from build123d import *

# Parameters (mm, degrees)
F_1_4_20_TAPPED_HOLE1_D     = 5.1054
F_1_4_20_TAPPED_HOLE1_DEPTH = 16.51
F_1_4_20_TAPPED_HOLE1_TIP   = 1.533816902
CUT_EXTRUDE1_DEPTH          = 9.525


with BuildPart() as part:
    # Sketch1 → Revolve2 (revolve)
    with BuildSketch(Plane(origin=(0, 0, 0), x_dir=(0, 0, -1), z_dir=(1, 0, 0)), mode=Mode.PRIVATE) as revolve2_sk:
        Polygon((38.1, 6.2865), (0, 6.2865), (0, 0), (82.55, 0), (82.55, 6.35), (44.45, 6.35), (44.45, 11.43), (38.1, 11.43), align=None)
    revolve(revolve2_sk.sketch.rotate(Axis((0, 0, 0), (0, 0, -1)), 90), axis=Axis((0, 0, 0), (0, 0, -1)))

    # 1/4-20 Tapped Hole1
    with Locations(Plane(origin=(0, 0, -82.55), x_dir=(-1, 0, 0), z_dir=(0, 0, -1))):
        with Locations((0, 0)):
            Hole(F_1_4_20_TAPPED_HOLE1_D / 2, depth=F_1_4_20_TAPPED_HOLE1_DEPTH)
            with Locations((0, 0, -(F_1_4_20_TAPPED_HOLE1_DEPTH + F_1_4_20_TAPPED_HOLE1_TIP / 2))):  # 118° drill point
                Cone(0, F_1_4_20_TAPPED_HOLE1_D / 2, F_1_4_20_TAPPED_HOLE1_TIP, mode=Mode.SUBTRACT)

    # Sketch4 → Cut-Extrude1 (cut)
    with BuildSketch(Plane.XY):
        with BuildLine():
            ThreePointArc((2.9407768, 5.55625), (0, 6.2865), (-2.9407768, 5.55625))
            Line((-2.9407768, 5.55625), (2.9407768, 5.55625))
        make_face()
        with BuildLine():
            ThreePointArc((6.28224205, 0.231337584), (5.444268701, 3.14325), (3.34146525, 5.324912416))
            Line((3.34146525, 5.324912416), (6.28224205, 0.231337584))
        make_face()
        with BuildLine():
            Line((6.28224205, -0.231337584), (3.34146525, -5.324912416))
            ThreePointArc((3.34146525, -5.324912416), (5.444268701, -3.14325), (6.28224205, -0.231337584))
        make_face()
        with BuildLine():
            Line((2.9407768, -5.55625), (-2.9407768, -5.55625))
            ThreePointArc((-2.9407768, -5.55625), (0, -6.2865), (2.9407768, -5.55625))
        make_face()
        with BuildLine():
            Line((-3.34146525, -5.324912416), (-6.28224205, -0.231337584))
            ThreePointArc((-6.28224205, -0.231337584), (-5.444268701, -3.14325), (-3.34146525, -5.324912416))
        make_face()
        with BuildLine():
            ThreePointArc((-3.34146525, 5.324912416), (-5.444268701, 3.14325), (-6.28224205, 0.231337584))
            Line((-6.28224205, 0.231337584), (-3.34146525, 5.324912416))
        make_face()
    extrude(amount=-CUT_EXTRUDE1_DEPTH, mode=Mode.SUBTRACT)


solid = part.part
Source: CAD feature listing. Evaluate the final solid. Frame: model axes, mm. A direction names the side the tool comes from. Round coordinates to 2 decimals unless told otherwise and drop trailing zeros. Loops run counter-clockwise (first coordinate to the right, second up) from the corner with the lowest first, then second, coordinate; pieces in that order, holes last.
Q1. Ray query, line 1 (Y direction, x = 0, z = -77); line 2 (Z direction, x = -7, y = 0.75); line 3 (X direction, y = 5.75, z = -13). Return the intervals inside material, ascending.
Q2. First-contact query: P1, Ø3, axis at x = 6.5, z = -41.5, coming from the +Y side; P2, Ø1.5, axis at x = -1.5, z = -10, coming from the -Y side; P3, Ø3, axis at y = -6, z = -13.5, coming from the +X side. Flat tips, straight axial feed; report the tip coordinate or a pass-through.
Q3. Section A-A, the plane z = -57. Return loops of the section in (x, y), plus the area to 3 significant figures.
Q4. Access query for faces 1 (the face through (5, 3, -9.525)), 2 (the face through (-5, -3, -9.525)), 3 (the face through (5, 5, -38.1)), 4 (the face through (0, -5.556, -5)), 5 (the face through (5, -3, -9.525)). Directions: +Z, -Z, +X, -X, +Y, -Y. A direction counts if a zero-diameter tool reaches every point of the face in a straight line with its end or side. Return the directions, or none.
Q5. Section B-B, the plane x = 4.75. Return loops of the section in (y, z) (3 decimals), plus the area to 3 significant figures.
Q6. Section D-D, the plane z = -30.5. Return loops of the section in (x, y).
Q7. Mould query, pull axis Y, two halves, no side actions, for faces 6 (the face through (2.435, 0.767, -74.179)), 7 (the face through (4.832, -2.742, -4.696)), 8 (the face through (0, 0, 0)). Classes: pulls with the +Y half, pulls with the -Y half, needs draft (parallel to the pull), parting line crosses it, or undercut.
Q8. Section C-C, the plane y = 8.25. Return loops of the section in (x, z), plus the area to 3 significant figures.
Solutions:
1. line 1: y = -6.35 to -2.55, 2.55 to 6.35
1. line 2: z = -44.45 to -38.1
1. line 3: x = -2.54 to 2.54
2. P1: stops at y = 10.28
2. P2: stops at y = -6.24
2. P3: stops at x = 4.39
3. outline: circle Ø12.7 at (0, 0)
3. area: 127 mm2
4. face 1: +Z, +X, +Y
4. face 2: +Z, -X, -Y
4. face 3: +Z
4. face 4: +Z, +X, -X, -Y
4. face 5: +Z, +X, -Y
5. outline: (-10.396, -44.45) - (-4.214, -44.45) - (-4.214, -82.55) - (4.214, -82.55) - (4.214, -44.45) - (10.396, -44.45) - (10.396, -38.1) - (4.118, -38.1) - (4.118, -9.525) - (2.885, -9.525) - (2.885, 0) - (-2.885, 0) - (-2.885, -9.525) - (-4.118, -9.525) - (-4.118, -38.1) - (-10.396, -38.1) - close
5. area: 743 mm2
6. outline: circle Ø12.57 at (0, 0)
7. face 6: undercut
7. face 7: pulls with the -Y half
7. face 8: needs draft
8. outline: (-7.91, -44.45) - (7.91, -44.45) - (7.91, -38.1) - (-7.91, -38.1) - close
8. area: 100 mm2
